from build123d import *

# Parameters (mm, degrees)
SKETCH1_R                            = 75.692
SKETCH1_R_2                          = 69.342
BOSS_EXTRUDE1_DEPTH                  = 22.225
SKETCH2_R                            = 75.692
BOSS_EXTRUDE2_DEPTH                  = 12.7
TAP_DRILL_FOR_1_4_20_TAP1_AT_2_COUNT = 2
TAP_DRILL_FOR_1_4_20_TAP1_AT_2_PITCH = 53.488399339
CIRPATTERN1_COUNT                    = 6


with BuildPart() as part:
    # Sketch1 → Boss-Extrude1 (new body)
    with BuildSketch(Plane(origin=(0, 0, 0), x_dir=(1, 0, 0), z_dir=(0, 1, 0))):
        Circle(SKETCH1_R)
        Circle(SKETCH1_R_2, mode=Mode.SUBTRACT)
    extrude(amount=BOSS_EXTRUDE1_DEPTH)

    # Sketch2 → Boss-Extrude2 (add)
    with BuildSketch(Plane.XZ):
        Circle(SKETCH2_R)
    extrude(amount=BOSS_EXTRUDE2_DEPTH)

    # Sketch4 → Tap Drill for 1/4-20 Tap1 (revolve, cut)
    with BuildSketch(Plane(origin=(73.997176623, 4.896298223, 15.927859738), x_dir=(0.210429897, 0, -0.97760895), z_dir=(0, 1, 0))):
        Polygon((0, 0), (0, 11.185816902), (2.5527, 9.652), (2.5527, 0), align=None)
    tap_drill_for_1_4_20_tap1 = revolve(axis=Axis((80.204993454, 4.896298223, 17.264089582), (-0.97760895, 0, -0.210429897)), mode=Mode.SUBTRACT)

    # Tap Drill for 1/4-20 Tap1 at 2: Tap Drill for 1/4-20 Tap1 ×2
    with Locations(*[Vector(-0.110438581, 0.851210999, 0.51307227) * (i * TAP_DRILL_FOR_1_4_20_TAP1_AT_2_PITCH) for i in range(1, TAP_DRILL_FOR_1_4_20_TAP1_AT_2_COUNT)]):
        add(tap_drill_for_1_4_20_tap1, mode=Mode.SUBTRACT)

    # CirPattern1: Tap Drill for 1/4-20 Tap1 ×6 about axis
    cirpattern1_axis = Axis((0, 22.225, 0), (0, -1, 0))
    for i in range(1, CIRPATTERN1_COUNT):
        add(tap_drill_for_1_4_20_tap1.rotate(cirpattern1_axis, i * 360 / CIRPATTERN1_COUNT), mode=Mode.SUBTRACT)

    # CirPattern1 copy 1 sketch → CirPattern1 copy 1 (revolve, cut)
    with BuildSketch(Plane(origin=(-3.515628412, 50.426212075, 80.653301416), x_dir=(0.951849134, 0, -0.306566839), z_dir=(0, 1, 0))):
        Polygon((0, 0), (0, 11.185816902), (2.5527, 9.652), (2.5527, 0), align=None)
    revolve(axis=Axis((-1.568928987, 50.426212075, 86.697543415), (-0.306566839, 0, -0.951849134)), mode=Mode.SUBTRACT)

    # CirPattern1 copy 2 sketch → CirPattern1 copy 2 (revolve, cut)
    with BuildSketch(Plane(origin=(-71.605622131, 50.426212075, 37.282027193), x_dir=(0.741419237, 0, 0.671042111), z_dir=(0, 1, 0))):
        Polygon((0, 0), (0, 11.185816902), (2.5527, 9.652), (2.5527, 0), align=None)
    revolve(axis=Axis((-75.866739537, 50.426212075, 41.990039348), (0.671042111, 0, -0.741419237)), mode=Mode.SUBTRACT)

    # CirPattern1 copy 3 sketch → CirPattern1 copy 3 (revolve, cut)
    with BuildSketch(Plane(origin=(-68.089993719, 50.426212075, -43.371274223), x_dir=(-0.210429897, 0, 0.97760895), z_dir=(0, 1, 0))):
        Polygon((0, 0), (0, 11.185816902), (2.5527, 9.652), (2.5527, 0), align=None)
    revolve(axis=Axis((-74.29781055, 50.426212075, -44.707504067), (0.97760895, 0, 0.210429897)), mode=Mode.SUBTRACT)

    # CirPattern1 copy 4 sketch → CirPattern1 copy 4 (revolve, cut)
    with BuildSketch(Plane(origin=(3.515628412, 50.426212075, -80.653301416), x_dir=(-0.951849134, 0, 0.306566839), z_dir=(0, 1, 0))):
        Polygon((0, 0), (0, 11.185816902), (2.5527, 9.652), (2.5527, 0), align=None)
    revolve(axis=Axis((1.568928987, 50.426212075, -86.697543415), (0.306566839, 0, 0.951849134)), mode=Mode.SUBTRACT)

    # CirPattern1 copy 5 sketch → CirPattern1 copy 5 (revolve, cut)
    with BuildSketch(Plane(origin=(71.605622131, 50.426212075, -37.282027193), x_dir=(-0.741419237, 0, -0.671042111), z_dir=(0, 1, 0))):
        Polygon((0, 0), (0, 11.185816902), (2.5527, 9.652), (2.5527, 0), align=None)
    revolve(axis=Axis((75.866739537, 50.426212075, -41.990039348), (-0.671042111, 0, 0.741419237)), mode=Mode.SUBTRACT)


solid = part.part
Input: part model. Units: mm. Frame: model coordinates. A direction names the side the tool comes from. Give positions to 0.01 mm unless a question says otherwise; leave off trailing zeros. Write each loop counter-clockwise with the first axis right and the second up, starting at its lowest first coordinate (ties: lowest second). Pieces come first, ordered by that corner, then holes. Notation, with made-up numbers: (38, -34.75) -> (48, -34.75) arc R30 ccw to (48, -2.75) -> close; hole circle Ø2 at (60.25, 46.25). An arc over 180 degrees is marked (long way). Use one line per item in the form item = value. Start each with the question number.
1) Set-up query: faces 1 (the cylindrical face through (23.54, 2.74, 68.62)), 2 (the cylindrical face through (-69.275, 10.957, -3.049)). Return all of +Z, -Z, +X, -X, +Y, -Y with unobstructed straight access to the full face (end or side cutting, diameter ignored); none if empty.
2) Section query B-B on z = 0. Return the cut outline in (x, y) (3 decimals), then the cut area to 3 significant figures.
3) Ray query, probe 1 along Z at (x, y) = (0, 13); probe 2 along Y at (x, z) = (49.5, 4.5). Return the intervals inside material, ascending. Write a range as from..to.
4) Section query A-A on x = 0. Return the cut outline in (y, z) (3 decimals), then the cut area to 3 significant figures.
5) Pin query (flat end, axial travel): pin 1 (10 mm diameter, centred on x = -60.5, y = -3, fed in from +Z); pin 2 (10 mm diameter, centred on x = 53.5, z = 13.5, fed in from +Y); pin 3 (1 mm diameter, centred on y = 10.5, z = 7.5, fed in from -X). Return the tip coordinate at first contact, or that it passes through.
6) Section query D-D on y = -3. Return the cut outline in (x, z).
7) Draft query along Y for faces 3 (the flat face through (33.3, 22.225, 61.3)), 4 (the cylindrical face through (-71.203, 2.744, -13.923)), 5 (the cylindrical face through (-20.45, 3.17, -69.62)), 6 (the flat face through (-1, -12.7, 1)). Return one class per face: pulls with the +Y half, pulls with the -Y half, needs draft (parallel to the pull), parting line crosses it, or undercut.
8) Section query C-C on y = 16. Return the cut outline in (x, z), then the cut area to 3 significant figures.
Outcome:
q1.face_1 = none
q1.face_2 = +Y
q2.outline = (-75.692, -12.7) -> (75.692, -12.7) -> (75.692, 22.225) -> (69.342, 22.225) -> (69.342, 0) -> (-69.342, 0) -> (-69.342, 22.225) -> (-75.692, 22.225) -> close
q2.area = 2,200 mm^2
q3.probe_1 = -75.69..-69.34, 69.34..75.69
q3.probe_2 = -12.7..0
q4.outline = (-12.7, -75.692) -> (22.225, -75.692) -> (22.225, -69.342) -> (0, -69.342) -> (0, 69.342) -> (22.225, 69.342) -> (22.225, 75.692) -> (-12.7, 75.692) -> close
q4.area = 2,200 mm^2
q5.pin_1 = 51.47
q5.pin_2 = 0
q5.pin_3 = -75.37
q6.outline = circle Ø151.38 at (0, 0)
q7.face_3 = pulls with the +Y half
q7.face_4 = undercut
q7.face_5 = undercut
q7.face_6 = pulls with the -Y half
q8.outline = circle Ø151.38 at (0, 0); hole circle Ø138.68 at (0, 0)
q8.area = 2,890 mm^2
